Source: three-view drawing plus pictorial views. Frame: mm from the lowest corner of the part. Give positions to 0.01 mm unless a question says otherwise; leave off trailing zeros. Loops run counter-clockwise (first coordinate to the right, second up) from the corner with the lowest first, then second, coordinate; pieces in that order, holes last.
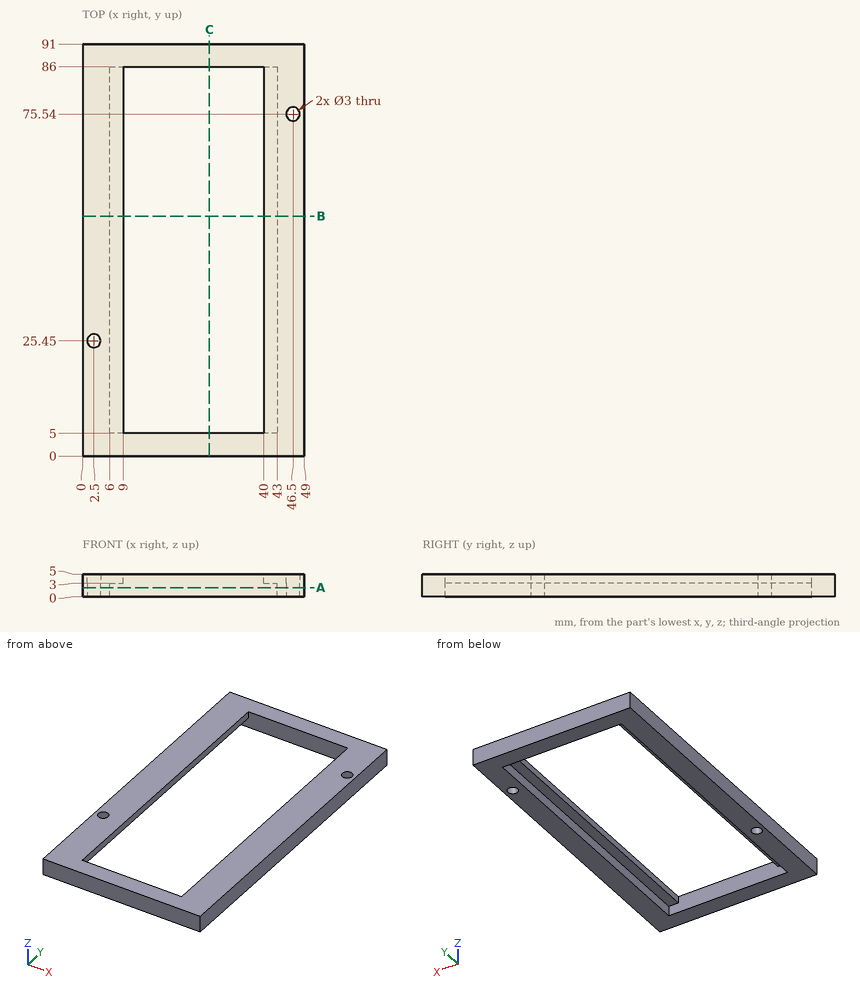
Q1. Pin query (flat end, axial travel): pin 1 Ø1.8 at (x, y) = (46.5, 75.54) entering from -Z; pin 2 Ø2.5 at (x, y) = (7.5, 30) entering from -Z. Return the tip coordinate at first contact, or that it passes through.
Q2. Section query B-B, the plane y = 53. Return loops of the section in (x, z).
Q3. Material intervals for probe 1 along X at (y, z) = (25.45, 2.25); probe 2 along X at (y, z) = (75.54, 2.15); probe 3 along X at (y, z) = (10.5, 3.2), sorted ascending.
Q4. Section query C-C, the plane x = 28. Return loops of the section in (y, z).
Q5. Section query A-A, the plane z = 2. Return loops of the section in (x, y), and give its area (3 significant figures).
Resolved:
1. pin 1: passes through
1. pin 2: stops at z = 3
2. outline: (0, 0) - (6, 0) - (6, 3) - (9, 3) - (9, 5) - (0, 5) - close; (40, 3) - (43, 3) - (43, 0) - (49, 0) - (49, 5) - (40, 5) - close
3. probe 1: x = 0 to 1, 4 to 6, 43 to 49
3. probe 2: x = 0 to 6, 43 to 45, 48 to 49
3. probe 3: x = 0 to 9, 40 to 49
4. outline: (0, 0) - (5, 0) - (5, 5) - (0, 5) - close; (86, 0) - (91, 0) - (91, 5) - (86, 5) - close
5. outline: (0, 0) - (49, 0) - (49, 91) - (0, 91) - close; hole circle Ø3 at (2.5, 25.45); hole (6, 5) - (43, 5) - (43, 86) - (6, 86) - close; hole circle Ø3 at (46.5, 75.54)
5. area: 1,450 mm2
